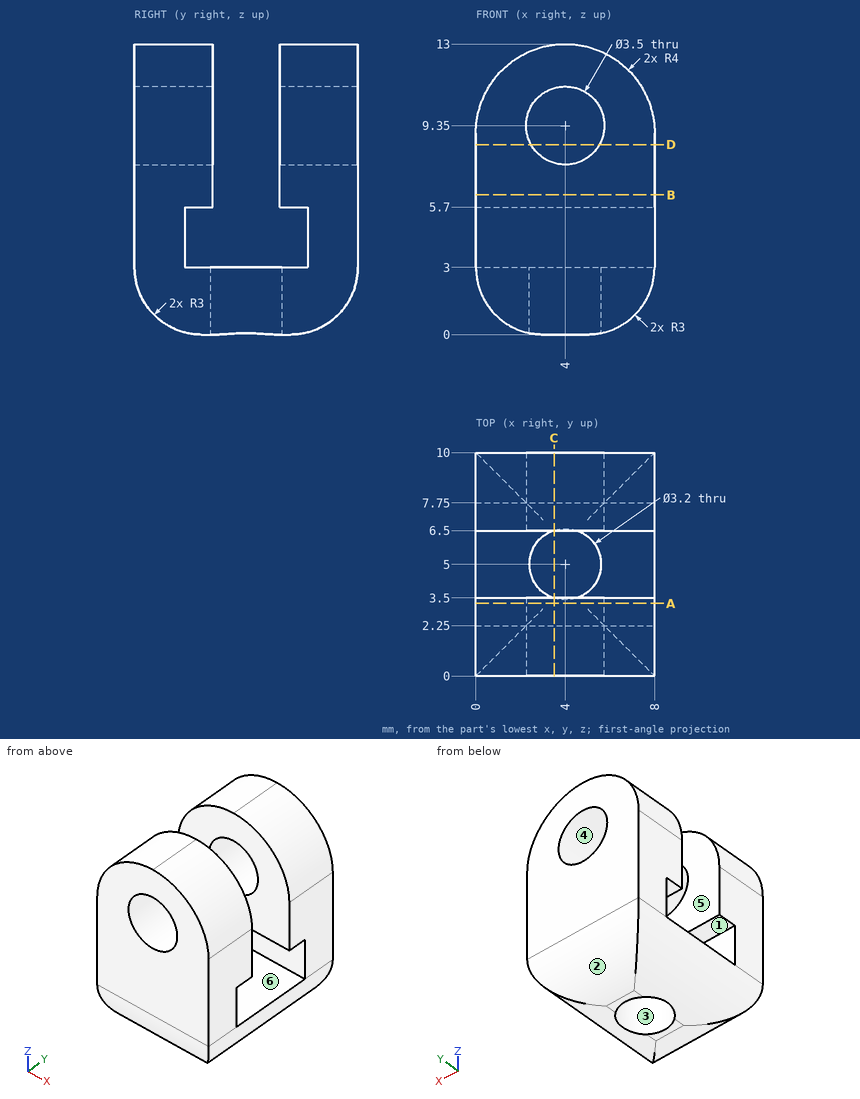
Geometry: see drawing. Coordinates: mm, zero at the bounding-box minimum. A direction names the side the tool comes from. Round coordinates to 2 decimals unless told otherwise and drop trailing zeros. Write each loop counter-clockwise with the first axis right and the second up, starting at its lowest first coordinate (ties: lowest second). Pieces come first, ordered by that corner, then holes.
Item 1: Section query C-C (x = 3.5). Return loops of the section in (y, z).
Item 2: Section query B-B (z = 6.25). Return loops of the section in (x, y), plus the area to 3 significant figures.
Item 3: Section query D-D (z = 8.5). Return loops of the section in (x, y).
Item 4: Material intervals for L1, parallel to Y at x = 6, z = 7.5; L2, parallel to Z at x = 5.5, y = 2.5; L3, parallel to Z at x = 3.25, y = 9, sorted ascending.
Item 5: Section query A-A (y = 3.25). Give the number of separate pieces and of enclosed holes in the cut face.
Item 6: Mould query, pull axis Z, two halves, no side actions, for the marked faces 1, 2 and 3. Classes: +Z half, -Z half, draft (parallel to the pull), parting line (faces both ways), or undercut.
Item 7: Set-up query: the marked faces 4, 5 and 6. Return all of +Z, -Z, +X, -X, +Y, -Y with unobstructed straight access to the full face (end or side cutting, diameter ignored); none if empty.
Item 8: Pin query (flat end, axial travel): P1, Ø1.5, axis at x = 1, y = 3.5, coming from the +Z side; P2, Ø1, axis at x = 3, y = 1, coming from the +Z side. Return the tip coordinate at first contact, or that it passes through.
Completed:
1. outline: (0, 3) arc R3 ccw to (3, 0) - (3.48, 0) - (3.48, 3) - (2.25, 3) - (2.25, 5.7) - (3.5, 5.7) - (3.5, 7.67) - (0, 7.67) - close; (0, 11.03) - (3.5, 11.03) - (3.5, 12.97) - (0, 12.97) - close; (6.5, 5.7) - (7.75, 5.7) - (7.75, 3) - (6.52, 3) - (6.52, 0) - (7, 0) arc R3 ccw to (10, 3) - (10, 7.67) - (6.5, 7.67) - close; (6.5, 11.03) - (10, 11.03) - (10, 12.97) - (6.5, 12.97) - close
2. outline: (0, 0) - (8, 0) - (8, 3.5) - (0, 3.5) - close; (0, 6.5) - (8, 6.5) - (8, 10) - (0, 10) - close
2. area: 56.0 mm2
3. outline: (0, 0) - (2.47, 0) - (2.47, 3.5) - (0, 3.5) - close; (0, 6.5) - (2.47, 6.5) - (2.47, 10) - (0, 10) - close; (5.53, 0) - (8, 0) - (8, 3.5) - (5.53, 3.5) - close; (5.53, 6.5) - (8, 6.5) - (8, 10) - (5.53, 10) - close
4. L1: y = 0 to 3.5, 6.5 to 10
4. L2: z = 0.04 to 3, 5.7 to 8.45, 10.25 to 12.71
4. L3: z = 0.76 to 7.77, 10.93 to 12.93
5. separate pieces: 2
5. enclosed holes: 1
6. face 1: undercut
6. face 2: -Z half
6. face 3: draft
7. face 4: +Y, -Y
7. face 5: +Z, +X, -X
7. face 6: +X, -X
8. P1: stops at z = 12.31
8. P2: stops at z = 12.97
